Input: dimensioned drawing with shaded views. Units: mm. Origin: part minimum x, y, z. Coordinates: 2 decimals unless noted, no trailing zeros. Loops run counter-clockwise (first coordinate to the right, second up) from the corner with the lowest first, then second, coordinate; pieces in that order, holes last. Notation, with made-up numbers: M 47.25,10 L 77.25,10 A19 ccw 77.25,46 Z; hole C 16,61.5 d5. An arc over 180 degrees is marked long. Write item = value, one per line. Start each with the question number.
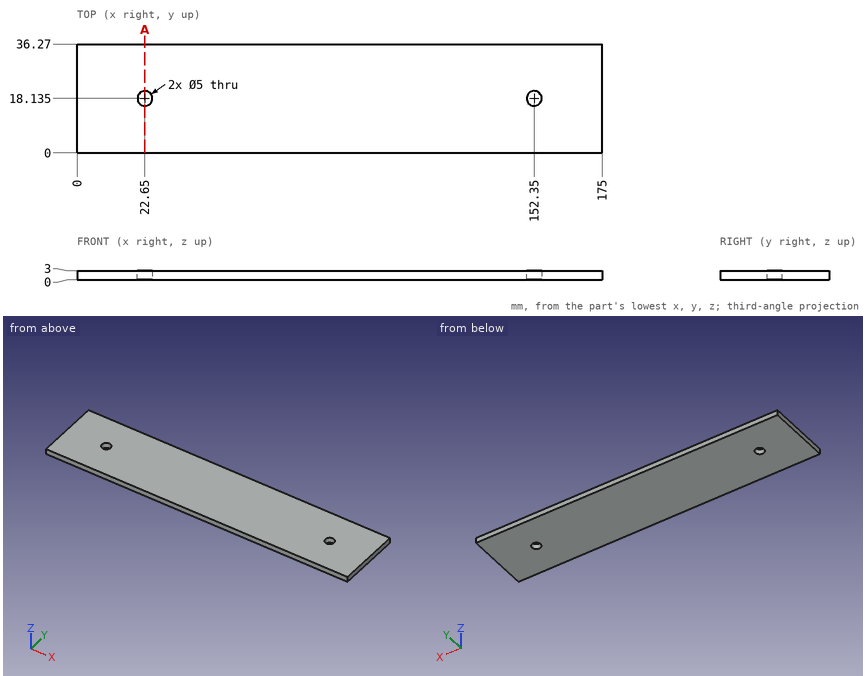
Item 1: Section query A-A (x = 22.65). Return the cut outline in (y, z) (3 decimals).
Item 2: First-contact query: pin 1 (8 mm diameter, centred on x = 70, y = 30, fed in from -Z). Flat tip, straight axial feed; report the tip coordinate or a pass-through.
Item 3: Line query: line 1 (Y direction, x = 152.35, z = 0.9) (3 decimals); line 2 (X direction, y = 16, z = 0.35); line 3 (X direction, y = 17.5, z = 2.7). Output: solid intervals per line, ascending. Write a range as from..to.
Verdict:
q1.outline = M 0,0 L 15.635,0 L 15.635,3 L 0,3 Z; M 20.635,0 L 36.27,0 L 36.27,3 L 20.635,3 Z
q2.pin_1 = 0
q3.line_1 = 0..15.635, 20.635..36.27
q3.line_2 = 0..21.35, 23.95..151.05, 153.65..175
q3.line_3 = 0..20.23, 25.07..149.93, 154.77..175
